Verification items for this drawing (mm, ordinates from the low corner). A direction names the side the tool comes from. Coordinates: 2 decimals unless noted, no trailing zeros. Write each loop counter-clockwise with the first axis right and the second up, starting at its lowest first coordinate (ties: lowest second). Pieces come first, ordered by that corner, then holes. Notation, with made-up numbers: M -0.75,49.25 L 49.25,49.25 A24 ccw 49.25,70.25 Z; hole C 87,49 d4. An arc over 180 degrees is marked long. Answer as CSV lines item,"result". Start each with the question number.
1) Material ranges on L1, parallel to Z at x = 16, y = 2.65; L2, parallel to Z at x = 7.25, y = 2.75 (1 decimal); L3, parallel to X at y = 3.45, z = 9, recorded low to high. Write a range as [from, to].
2) Go/stop test with flat-tipped pins: pin 1 Ø4 at (x, z) = (17, 6.5) entering from +Y; pin 2 Ø1.3 at (x, z) = (16, 12.5) entering from -Y; pin 3 Ø2 at (y, z) = (1.5, 4.5) entering from -X. Record where each tip stops, or that it passes through.
3) Access from +Z, -Z, +X, -X, +Y, -Y to the whole of each face (thin tool, end or side, straight path). Record for the marked faces 5, 6 and 7.
4) Draft check along Z on the marked faces 1, 2, 3 and 4. Enter one of: +Z half, -Z half, draft (parallel to the pull), parting line (faces both ways), or undercut.
5) Section check B-B (x = 16). Record the cut outline in (y, z).
6) Section check A-A (y = 1.7). State how many separate pieces and enclosed holes the cut face has, and give its area (3 significant figures).
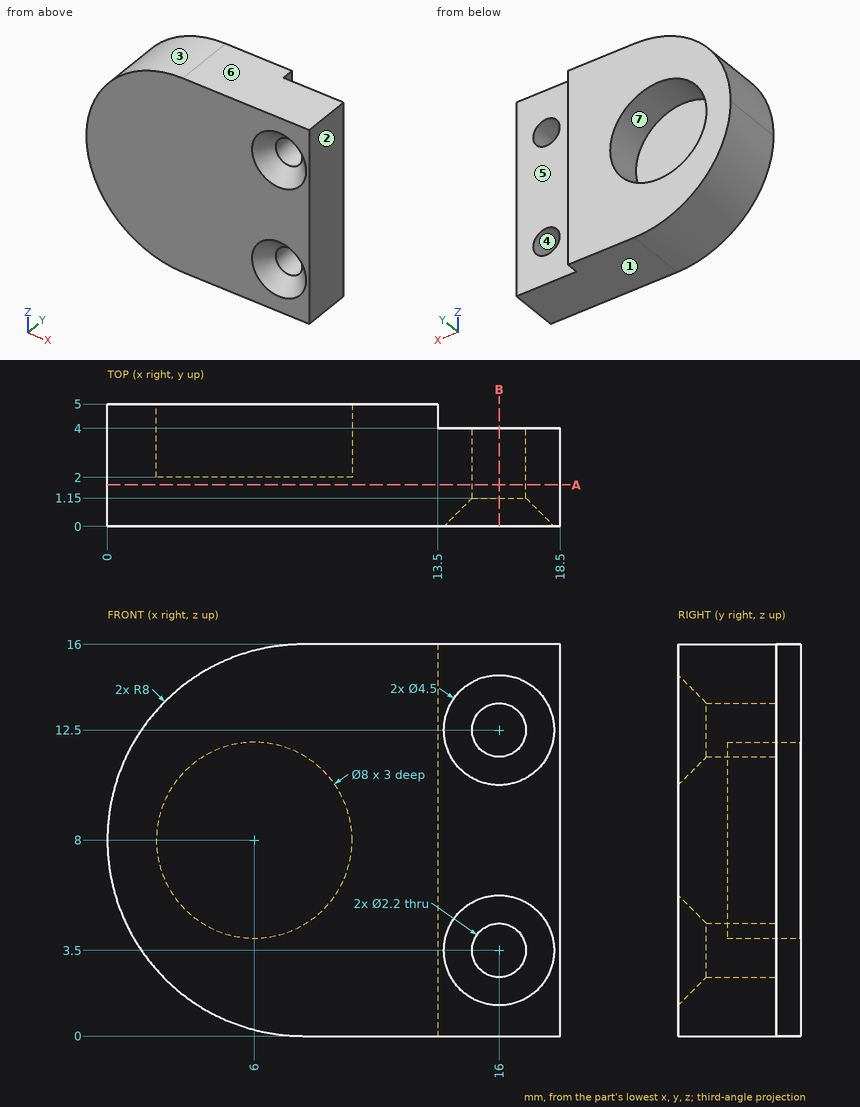
Results found:
1,L1,"z = [0, 2.4], [4.6, 11.4], [13.6, 16]"
1,L2,"z = [0, 4.2], [11.8, 16]"
1,L3,"x = [0.06, 2.13], [9.87, 18.5]"
2,pin 1,"stops at y = 4"
2,pin 2,"passes through"
2,pin 3,"stops at x = 0.4"
3,face 5,"+Z, -Z, +X, +Y"
3,face 6,"+Z, +X, -X, +Y, -Y"
3,face 7,"+Y"
4,face 1,"-Z half"
4,face 2,"draft"
4,face 3,"+Z half"
4,face 4,"undercut"
5,outline,"M 0,0 L 4,0 L 4,2.4 L 1.15,2.4 L 0,1.25 Z; M 0,5.75 L 1.15,4.6 L 4,4.6 L 4,11.4 L 1.15,11.4 L 0,10.25 Z; M 0,14.75 L 1.15,13.6 L 4,13.6 L 4,16 L 0,16 Z"
6,separate pieces,"1"
6,enclosed holes,"2"
6,area,"261 mm2"
